```python
from build123d import *

# Parameters (mm, degrees)
F0_W     = 76.2
F0_H     = 63.462952
F1_DEPTH = 38.1
F2_T     = -3.96875
F3_W     = 59.153464
F3_H     = 3.775753
F4_DEPTH = 84.455
F5_W     = 8.255
F5_H     = 8.262471
F5_W_2   = 6.50875
F5_H_2   = 6.35
F6_DEPTH = 6.35
F8_W     = 52.838832
F8_H     = 26.304427
F9_DEPTH = 6.35


with BuildPart() as f1:
    # F0 (on Top) → F1 (new body)
    with BuildSketch(Plane.XY):
        with Locations((6.831993, -1.102022)):
            Rectangle(F0_W, F0_H)
    extrude(amount=F1_DEPTH)

    # F2
    f2_openings = [f1.faces().sort_by_distance(p)[0] for p in [
        (6.831993, -1.102022, 38.1),
    ]]
    offset(amount=F2_T, openings=f2_openings)

    # F3 (on face) → F4 (cut)
    with BuildSketch(Plane.YZ.offset(44.931993)):
        with Locations((-0.988886, 33.613619)):
            Rectangle(F3_W, F3_H)
    extrude(amount=-F4_DEPTH, mode=Mode.SUBTRACT)

    # F5 (on face) → F6 (cut)
    with BuildSketch(Plane.YZ.offset(44.931993)):
        with Locations((13.865454, 10.481236)):
            Rectangle(F5_W, F5_H)
        with Locations((-5.635625, 9.525)):
            Rectangle(F5_W_2, F5_H_2)
    extrude(amount=-F6_DEPTH, mode=Mode.SUBTRACT)

    # F8 (on face) → F9 (cut)
    with BuildSketch(Plane(origin=(-31.268007, 0, 0), x_dir=(0, -1, 0), z_dir=(-1, 0, 0))):
        with Locations((1.379967, 18.573529)):
            Rectangle(F8_W, F8_H)
    extrude(amount=-F9_DEPTH, mode=Mode.SUBTRACT)


solid = f1.part
```
Can you work these out from the model? Positions are in its coordinate system, mm. A direction names the side the tool comes from. Round coordinates to 2 decimals unless told otherwise and drop trailing zeros. Loops run counter-clockwise (first coordinate to the right, second up) from the corner with the lowest first, then second, coordinate; pieces in that order, holes last. Notation, with made-up numbers: (6, -6.5) -> (34, -6.5) arc R26 ccw to (34, 8.5) -> close; hole circle Ø7 at (89, 27). An arc over 180 degrees is marked (long way). One line per item, written item: value. Start each with the question number.
1. For faces 1 (the flat face through (6, -1, 3.969)), 2 (the flat face through (-29, -27.799, 18)), 3 (the flat face through (43, -8.89, 9)), which set-ups out of +Z, -Z, +X, -X, +Y, -Y let a thin tool reach every point of the face, with its end or its side?
2. If we section it at D-D, the plane z = 28: Write out the boundary of the cut face in (x, y), then the cut area to 3 significant figures.
3. If we section it at B-B, the plane x = 39: Write out the boundary of the cut face in (y, z), then the cut area to 3 significant figures.
4. For pin 1 (1.5 mm diameter, centred on y = -20.5, z = 17.5, fed in from -X); pin 2 (6 mm diameter, centred on x = 27.5, y = -1.5, fed in from +Z); pin 3 (10 mm diameter, centred on x = -19, y = -3.5, fed in from -Z), each with a flat end and sliding along its axis, tell me the tip position at first contact or that it passes through.
5. If we section it at C-C, the plane y = 14: Write out the boundary of the cut face in (x, z), then the cut area to 3 significant figures.
6. If we section it at A-A, the plane y = -12.5: Write out the boundary of the cut face in (x, z), then the cut area to 3 significant figures.
7. If I drill on probe 1 along Y at (x, z) = (-27, 24.5); probe 2 along Y at (x, z) = (-23.5, 35); probe 3 along Z at (x, y) = (4.5, -29.5), over which ranges is the centre line in solid material (lowest first)?
8. If we mould it in two halves opening along Y, with no side actions, what happens to faces 4 (the flat face through (43, 14, 14.612)), 5 (the flat face through (6, -32.833, 19)), 6 (the flat face through (44.932, -2, 19))? For each: pulls with the +Y half, pulls with the -Y half, needs draft (parallel to the pull), parting line crosses it, or undercut.
Calculated:
1. face 1: +Z
1. face 2: -X
1. face 3: +X, -X
2. outline: (-31.27, -32.83) -> (44.93, -32.83) -> (44.93, 30.63) -> (-31.27, 30.63) -> (-31.27, 25.04) -> (-27.3, 25.04) -> (-27.3, 26.66) -> (40.96, 26.66) -> (40.96, -28.86) -> (-27.3, -28.86) -> (-27.3, -27.8) -> (-31.27, -27.8) -> close
2. area: 836 mm²
3. outline: (-32.83, 0) -> (30.63, 0) -> (30.63, 38.1) -> (26.66, 38.1) -> (26.66, 35.5) -> (28.59, 35.5) -> (28.59, 31.73) -> (26.66, 31.73) -> (26.66, 3.97) -> (-28.86, 3.97) -> (-28.86, 31.73) -> (-30.57, 31.73) -> (-30.57, 35.5) -> (-28.86, 35.5) -> (-28.86, 38.1) -> (-32.83, 38.1) -> close
3. area: 509 mm²
4. pin 1: stops at x = 40.96
4. pin 2: stops at z = 3.97
4. pin 3: stops at z = 0
5. outline: (-31.27, 0) -> (44.93, 0) -> (44.93, 6.35) -> (40.96, 6.35) -> (40.96, 3.97) -> (-27.3, 3.97) -> (-27.3, 5.42) -> (-31.27, 5.42) -> close; (-31.27, 35.5) -> (-27.3, 35.5) -> (-27.3, 38.1) -> (-31.27, 38.1) -> close; (40.96, 14.61) -> (44.93, 14.61) -> (44.93, 31.73) -> (40.96, 31.73) -> close; (40.96, 35.5) -> (44.93, 35.5) -> (44.93, 38.1) -> (40.96, 38.1) -> close
5. area: 406 mm²
6. outline: (-31.27, 0) -> (44.93, 0) -> (44.93, 31.73) -> (40.96, 31.73) -> (40.96, 3.97) -> (-27.3, 3.97) -> (-27.3, 5.42) -> (-31.27, 5.42) -> close; (-31.27, 35.5) -> (-27.3, 35.5) -> (-27.3, 38.1) -> (-31.27, 38.1) -> close; (40.96, 35.5) -> (44.93, 35.5) -> (44.93, 38.1) -> (40.96, 38.1) -> close
6. area: 439 mm²
7. probe 1: y = -32.83 to -28.86, 26.66 to 30.63
7. probe 2: y = -32.83 to -30.57, 28.59 to 30.63
7. probe 3: z = 0 to 31.73, 35.5 to 38.1
8. face 4: undercut
8. face 5: pulls with the -Y half
8. face 6: needs draft
